CAD build for the part. Positions are in the model's coordinates, mm. Coordinates: 2 decimals unless noted, no trailing zeros. Loops run counter-clockwise (first coordinate to the right, second up) from the corner with the lowest first, then second, coordinate; pieces in that order, holes last.
1) Wall check: line 1 along Z through (x, y) = (-120, -29); line 2 along X through (y, z) = (33, 304); line 3 along Y through (x, z) = (-366, 589.5). Give the ranges that are in metal, low to high.
2) Saw through at C-C, the plane x = 304. Write the cut outline in (y, z).
3) Pin check, flat tip, straight feed: pin 1 Ø1 at (x, y) = (77, 5.5) entering from +Z. Stop position of the tip, or through.
4) Saw through at A-A, the plane x = 2. Write the cut outline in (y, z).
5) Saw through at B-B, the plane z = 1049. Write the cut outline in (x, y), and give its area (3 significant figures).
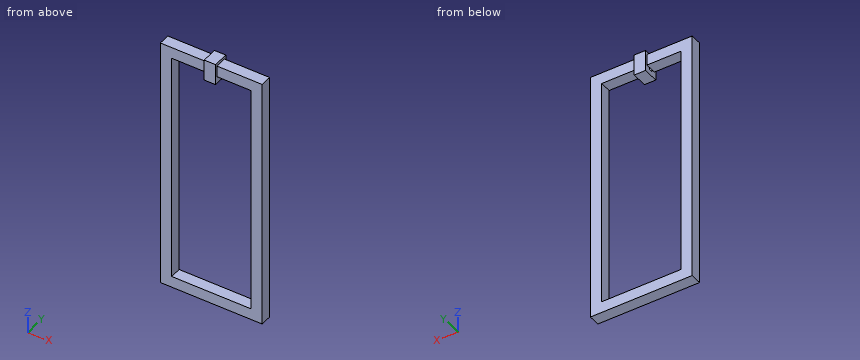
```python
from build123d import *

# Parameters (mm, degrees)
F0_W          = 914.4
F0_H          = 101.6
F1_DEPTH      = 2286
F2_T          = -101.6
F3_W          = 101.6
F3_H          = 139.7
F4_DEPTH      = 165.1
F4_DEPTH_BACK = 25.4
F5_T          = 50.8
F5_T3_DEPTH   = 203.2
F6_SIZE       = 5.08


# Not quite as in the source:
# - a shell that OpenCascade refuses in one call is made with other operations: the cavity is built on its own and cut out


with BuildPart() as f1:
    # F0 (on Top) → F1 (new body)
    with BuildSketch(Plane.XY):
        Rectangle(F0_W, F0_H)
    extrude(amount=F1_DEPTH)

    # F2
    f2_openings = [f1.faces().sort_by_distance(p)[0] for p in [
        (0, -50.8, 1143),
        (0, 50.8, 1143),
    ]]
    offset(amount=F2_T, openings=f2_openings)

    # F3 (on face) → F4 (join, two sides)
    with BuildSketch(Plane.XY.offset(2286)) as f4_sk:
        Rectangle(F3_W, F3_H)
    extrude(amount=-F4_DEPTH)
    extrude(f4_sk.sketch, amount=F4_DEPTH_BACK)

    # F5: shell of thickness 50.8, made by hand


with BuildPart() as f5_core1:
    # F5_t2: copy of F1
    add(f1.part)

    # the walls: a layer under each face that stays
    f5_faces = [f5_core1.faces().sort_by_distance(p)[0] for p in [
        (-457.2, 0, 1143),
        (391.8857142857, 50.8, 2122.7142857143),
        (-391.8857142857, -50.8, 2122.7142857143),
        (0, 0, 0),
        (-254, 0, 2286),
        (-203.2, 0, 2184.4),
        (-355.6, 0, 1143),
        (0, 0, 101.6),
        (355.6, 0, 1143),
        (203.2, 0, 2184.4),
        (254, 0, 2286),
        (457.2, 0, 1143),
        (0, 0, 2120.9),
        (0, 69.85, 2216.15),
        (0, -69.85, 2216.15),
        (0, 0, 2311.4),
    ]]
    thicken(f5_faces, amount=-F5_T, mode=Mode.SUBTRACT)

    # F5_s4 → F5_t3 (cut)
    with BuildSketch(Plane.XZ.offset(-101.6)):
        Polygon((-355.092, 2183.892), (-355.6, 2235.2), (-406.4, 2235.2), (-406.4, 2184.4), align=None)
        Polygon((-355.092, 102.108), (-406.4, 101.6), (-406.4, 50.8), (-355.6, 50.8), align=None)
        Polygon((355.092, 102.108), (355.6, 50.8), (406.4, 50.8), (406.4, 101.6), align=None)
        Polygon((355.092, 2183.892), (406.4, 2184.4), (406.4, 2235.2), (355.6, 2235.2), align=None)
    extrude(amount=F5_T3_DEPTH, mode=Mode.SUBTRACT)


with BuildPart() as f1_1:
    add(f1.part)

    # what is left inside the walls is the cavity
    f5_cavity = [f5_core1.part.solids().sort_by_distance(p)[0] for p in [
        (0, -18.542, 2201.333333),
    ]]
    add(f5_cavity, mode=Mode.SUBTRACT)

    # F6
    f6_edges = [f1_1.edges().sort_by_distance(p)[0] for p in [
        (-50.8, 0, 2171.7),
    ]]
    chamfer(f6_edges, length=F6_SIZE)


solid = f1_1.part
```
Data:
1. line 1: z = 0 to 101.6, 2184.4 to 2286
1. line 2: x = -457.2 to -355.6, 355.6 to 457.2
1. line 3: y = -50.8 to 50.8
2. outline: (-50.8, 0) - (50.8, 0) - (50.8, 101.6) - (-50.8, 101.6) - close; (-50.8, 2184.4) - (50.8, 2184.4) - (50.8, 2286) - (-50.8, 2286) - close
3. pin 1: stops at z = 2286
4. outline: (-69.85, 2120.9) - (69.85, 2120.9) - (69.85, 2311.4) - (-69.85, 2311.4) - close; (-50.8, 0) - (50.8, 0) - (50.8, 101.6) - (-50.8, 101.6) - close; hole (-19.05, 2171.7) - (19.05, 2171.7) - (19.05, 2260.6) - (-19.05, 2260.6) - close
5. outline: (-457.2, -50.8) - (-355.6, -50.8) - (-355.6, 50.8) - (-457.2, 50.8) - close; (355.6, -50.8) - (457.2, -50.8) - (457.2, 50.8) - (355.6, 50.8) - close
5. area: 20,600 mm2
